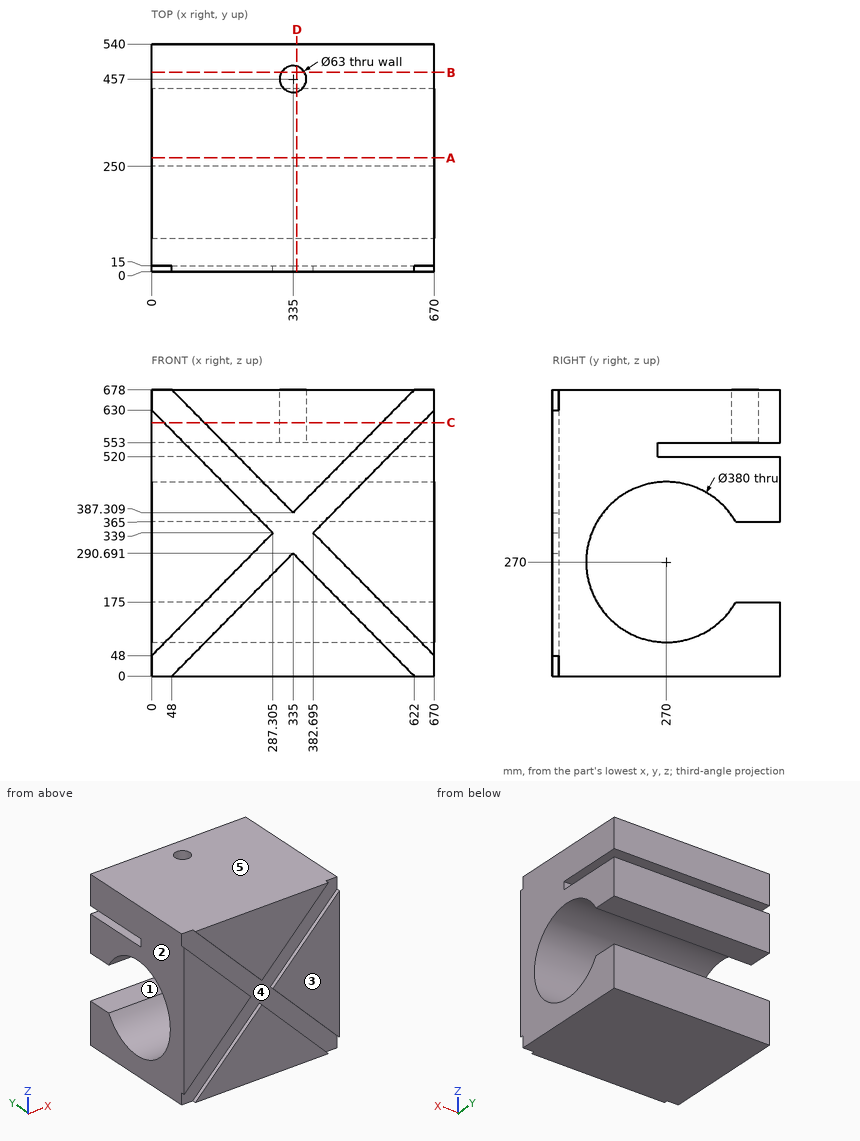
Geometry: see drawing. Coordinates: mm, zero at the bounding-box minimum. A direction names the side the tool comes from. Give positions to 0.01 mm unless a question says otherwise; leave off trailing zeros. Write each loop counter-clockwise with the first axis right and the second up, starting at its lowest first coordinate (ties: lowest second). Pieces come first, ordered by that corner, then holes. Notation, with made-up numbers: M 82.5,-15 L 114.5,-15 A35 cw 114.5,18 Z; hole C 49.25,30 d4. An arc over 180 degrees is marked long. Answer in a Markdown table with one row per item. Add a question column.
(1) Section D-D on x = 344. Return loops of the section in (y, z) (1 decimal), and give its area (3 significant figures).
(2) Reachability of the marked faces 1 and 2 from +Z, -Z, +X, -X, +Y, -Y: full face, straight path, thin tool, end or side. Return the list, or none.
(3) Mould query, pull axis Z, two halves, no side actions, for the marked faces 3, 4 and 5. Classes: +Z half, -Z half, draft (parallel to the pull), parting line (faces both ways), or undercut.
(4) Ray query, line 1 (Z direction, x = 124.5, y = 264) (1 decimal); line 2 (Z direction, x = 408.5, y = 270); line 3 (Y direction, x = 220, z = 270). Return the intervals inside material, ascending.
(5) Section B-B on y = 473. Return loops of the section in (x, z).
(6) First-contact query: pin 1 (12 mm diameter, centred on x = 466, z = 426.5, fed in from -Y); pin 2 (10 mm diameter, centred on x = 368, z = 341, fed in from +Y). Flat tips, straight axial feed; report the tip coordinate or a pass-through.
(7) Section C-C on z = 600.5. Return loops of the section in (x, y) (1 decimal), and give its area (3 significant figures).
(8) Section A-A on y = 270. Return loops of the section in (x, z).
Result set:
| question | item | result |
|---|---|---|
| 1 | outline | M 0,0 L 540,0 L 540,175 L 434.5,175 A190 cw long 434.5,365 L 540,365 L 540,520 L 250,520 L 250,553 L 426.8,553 L 426.8,678 L 0,678 L 0,396.4 L 15,396.4 L 15,281.6 L 0,281.6 Z; M 487.2,553 L 540,553 L 540,678 L 487.2,678 Z |
| 1 | area | 217,000 mm^2 |
| 2 | face 1 | +X, -X, +Y |
| 2 | face 2 | +Z, -Z, -X, +Y, -Y |
| 3 | face 3 | draft |
| 3 | face 4 | undercut |
| 3 | face 5 | +Z half |
| 4 | line 1 | z = 0 to 80.1, 459.9 to 520, 553 to 678 |
| 4 | line 2 | z = 0 to 80, 460 to 520, 553 to 678 |
| 4 | line 3 | y = 15 to 80 |
| 5 | outline | M 0,0 L 670,0 L 670,175 L 0,175 Z; M 0,365 L 670,365 L 670,520 L 0,520 Z; M 0,553 L 307.87,553 L 307.87,678 L 0,678 Z; M 362.13,553 L 670,553 L 670,678 L 362.13,678 Z |
| 6 | pin 1 | stops at y = 0 |
| 6 | pin 2 | stops at y = 95.86 |
| 7 | outline | M 0,0 L 29.1,0 L 29.1,15 L 124.5,15 L 124.5,0 L 545.5,0 L 545.5,15 L 640.9,15 L 640.9,0 L 670,0 L 670,540 L 0,540 Z; hole C 335,457 d63 |
| 7 | area | 356,000 mm^2 |
| 8 | outline | M 0,0 L 670,0 L 670,80 L 0,80 Z; M 0,460 L 670,460 L 670,520 L 0,520 Z; M 0,553 L 670,553 L 670,678 L 0,678 Z |
